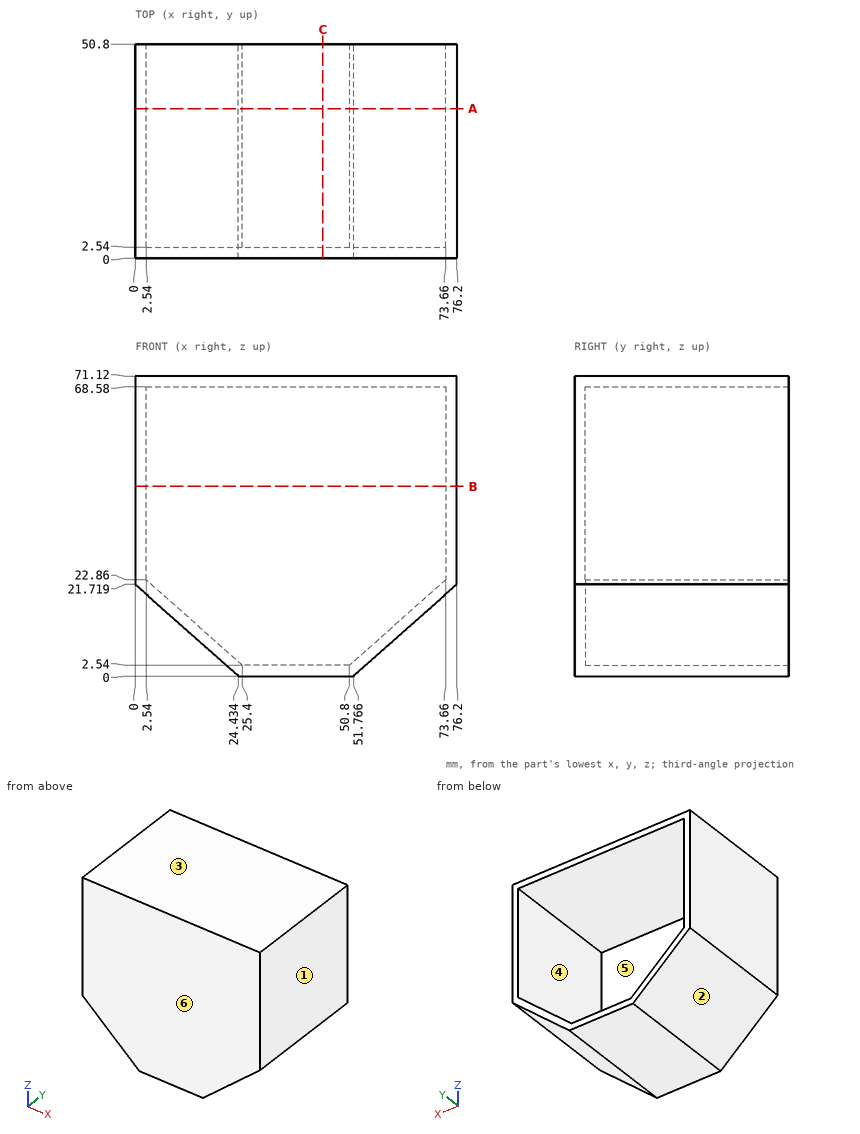
Here's the drawing with two shaded views (mm, measured from the low corner). I have some questions. A direction names the side the tool comes from. Coordinates: 2 decimals unless noted, no trailing zeros. Loops run counter-clockwise (first coordinate to the right, second up) from the corner with the lowest first, then second, coordinate; pieces in that order, holes last. Notation, with made-up numbers: M 58.25,73.5 L 84.25,73.5 A15 cw 84.25,77.5 Z; hole C -26,70.5 d3. An arc over 180 degrees is marked long. Answer as CSV lines item,"result". Start each with the question number.
1. Suppose I cut it at A-A, the plane y = 35.5. List the corners of the cut face in (x, z) for me (1 decimal).
2. For the marked faces 5 and 6, which set-ups out of +Z, -Z, +X, -X, +Y, -Y let a thin tool reach every point of the face, with its end or its side?
3. For pin 1 Ø3 at (x, z) = (29, 63.5) entering from +Y; pin 2 Ø1 at (y, z) = (6.5, 8.5) entering from +X, each with a flat end and sliding along its axis, tell me the tip position at first contact or that it passes through.
4. If I drill on probe 1 along Z at (x, y) = (35.5, 22.5); probe 2 along X at (y, z) = (29, 54.5); probe 3 along Y at (x, z) = (16.5, 31), over which ranges is the centre line in solid material (lowest first)? Write a range as [from, to].
5. Suppose I cut it at C-C, the plane x = 44.5. List the corners of the cut face in (y, z) for me, plus the area to 3 significant figures.
6. Suppose I cut it at B-B, the plane z = 45. List the corners of the cut face in (x, y) for me.
7. Thinking about a two-plate mould opening in Z: for the marked faces 1, 2, 3 and 4, which applies, +Z half, -Z half, draft (parallel to the pull), parting line (faces both ways), or undercut?
Output:
1,outline,"M 0,21.7 L 24.4,0 L 51.8,0 L 76.2,21.7 L 76.2,71.1 L 0,71.1 Z; hole M 2.5,22.9 L 25.4,2.5 L 50.8,2.5 L 73.7,22.9 L 73.7,68.6 L 2.5,68.6 Z"
2,face 5,"+Y"
2,face 6,"+Z, -Z, +X, -X, -Y"
3,pin 1,"stops at y = 2.54"
3,pin 2,"stops at x = 61.89"
4,probe 1,"z = [0, 2.54], [68.58, 71.12]"
4,probe 2,"x = [0, 2.54], [73.66, 76.2]"
4,probe 3,"y = [0, 2.54]"
5,outline,"M 0,0 L 50.8,0 L 50.8,2.54 L 2.54,2.54 L 2.54,68.58 L 50.8,68.58 L 50.8,71.12 L 0,71.12 Z"
5,area,"426 mm^2"
6,outline,"M 0,0 L 76.2,0 L 76.2,50.8 L 73.66,50.8 L 73.66,2.54 L 2.54,2.54 L 2.54,50.8 L 0,50.8 Z"
7,face 1,"draft"
7,face 2,"-Z half"
7,face 3,"+Z half"
7,face 4,"undercut"
